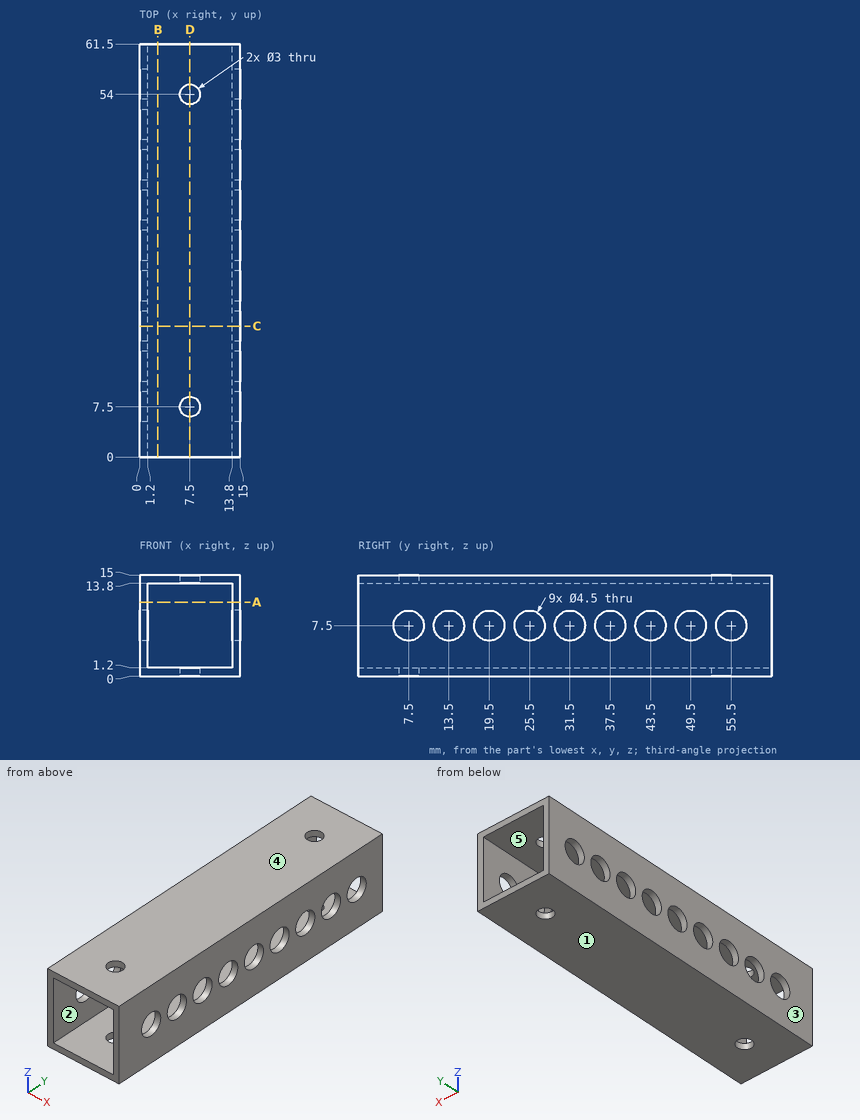
Geometry check sheet. Reference: drawing and pictorial views, mm from the part's lowest x, y, z. A direction names the side the tool comes from. Round coordinates to 2 decimals unless told otherwise and drop trailing zeros. Order: outer loops, then holes, each group sorted by start corner. A loop starts at its lowest first (then second) coordinate and runs counter-clockwise, first axis right, second up. Notation, with made-up numbers: (-12.75, -15) - (25.25, -15) arc R7 ccw to (25.25, -9) - close; hole circle Ø8 at (35, -36.5). An arc over 180 degrees is marked (long way). Use a Markdown table: item, result. Add a question column.
1) Section check B-B (x = 2.75). Record the cut outline in (y, z).
2) Thickness scan on line 1 along Y through (x, z) = (7.5, 14.45); line 2 along Z through (x, y) = (2.25, 28); line 3 along Z through (x, y) = (0.5, 49.5). Record the ranges inside material, lowest first.
3) Mould release check, pull along X, two halves, no side actions. Record for the marked faces 1, 2 and 3: released by +X, released by -X, zero draft, split by the parting line, or undercut.
4) Set-up check for the marked faces 4 and 5: record each of +Z, -Z, +X, -X, +Y, -Y from which the full face is reachable in a straight line by a thin tool's end or side.
5) Section check A-A (z = 11). Record the cut outline in (x, y).
6) Section check C-C (y = 19.5). Record the cut outline in (x, z).
7) Section check D-D (x = 7.5). Record the cut outline in (y, z), then the cut area to 3 significant figures.
8) Gauge pin test, flat end, axial feed: P1, Ø3.5, axis at y = 19.5, z = 7.5, coming from the +X side. Record the tip position at first contact, or that the pin passes through.
Established:
| question | item | result |
|---|---|---|
| 1 | outline | (0, 0) - (61.5, 0) - (61.5, 1.2) - (0, 1.2) - close; (0, 13.8) - (61.5, 13.8) - (61.5, 15) - (0, 15) - close |
| 2 | line 1 | 0 to 6, 9 to 52.5, 55.5 to 61.5 |
| 2 | line 2 | 0 to 1.2, 13.8 to 15 |
| 2 | line 3 | 0 to 5.25, 9.75 to 15 |
| 3 | face 1 | zero draft |
| 3 | face 2 | undercut |
| 3 | face 3 | released by -X |
| 4 | face 4 | +Z, +X, -X, +Y, -Y |
| 4 | face 5 | +Y, -Y |
| 5 | outline | (0, 0) - (1.2, 0) - (1.2, 61.5) - (0, 61.5) - close; (13.8, 0) - (15, 0) - (15, 61.5) - (13.8, 61.5) - close |
| 6 | outline | (0, 0) - (15, 0) - (15, 5.25) - (13.8, 5.25) - (13.8, 1.2) - (1.2, 1.2) - (1.2, 5.25) - (0, 5.25) - close; (0, 9.75) - (1.2, 9.75) - (1.2, 13.8) - (13.8, 13.8) - (13.8, 9.75) - (15, 9.75) - (15, 15) - (0, 15) - close |
| 7 | outline | (0, 0) - (6, 0) - (6, 1.2) - (0, 1.2) - close; (0, 13.8) - (6, 13.8) - (6, 15) - (0, 15) - close; (9, 0) - (52.5, 0) - (52.5, 1.2) - (9, 1.2) - close; (9, 13.8) - (52.5, 13.8) - (52.5, 15) - (9, 15) - close; (55.5, 0) - (61.5, 0) - (61.5, 1.2) - (55.5, 1.2) - close; (55.5, 13.8) - (61.5, 13.8) - (61.5, 15) - (55.5, 15) - close |
| 7 | area | 133 mm2 |
| 8 | P1 | through |
